from build123d import *


with BuildPart() as part:
    # Model → Повернуть1 (revolve)
    with BuildSketch(Plane.XY, mode=Mode.PRIVATE) as revolve_1_sk:
        Polygon((0, 0), (0, -22.297439151), (0.406986693, -22.5), (4.563171418, -22.5), (4.765560012, -22.297439151), (7.132579794, -17.847080181), (8.034078204, -18.53333859), (8.879510019, -18.045513069), (9.72476958, -18.601092135), (10.570023757, -18.045513069), (11.410266397, -18.530582514), (12.250724355, -18.045513069), (12.250724355, -17.741666414), (17.616266787, -17.741666414), (17.818865316, -17.539062501), (17.818865316, -16.425629172), (18.426031098, -16.425629172), (18.426031098, -17.387144556), (21.362129874, -17.387144556), (21.362129874, -16.425629172), (21.868225167, -16.425629172), (21.868225167, -17.493893941), (27.334902683, -17.493893941), (27.790688815, -18), (32.143900705, -18), (32.599331562, -17.544536845), (33.552402733, -17.544536845), (33.552338057, -16.75), (37.095113357, -16.75), (37.5, -16.425629172), (37.5, -12.801691559), (38.665364669, -12.801691559), (38.665364669, -13.294307916), (40.791343859, -13.294307916), (41.5, -12.586706835), (41.5, -10.75), (42.129406807, -10.75), (43.8, -9.548466361), (43.8, 0), align=None)
    revolve(revolve_1_sk.sketch.rotate(Axis((0, 0, 0), (1, 0, 0)), 270), axis=Axis((0, 0, 0), (1, 0, 0)))


solid = part.part
Part model, mm, in its own coordinate system. A direction names the side the tool comes from. Coordinates: 2 decimals unless noted, no trailing zeros. Write each loop counter-clockwise with the first axis right and the second up, starting at its lowest first coordinate (ties: lowest second). Pieces come first, ordered by that corner, then holes. Notation, with made-up numbers: (27, -32.5) - (41, -32.5) arc R27 cw to (41, -12.5) - close; hole circle Ø9 at (-1, 48). An arc over 180 degrees is marked (long way). Put each result on its own line as item: value.
1. Two-plate mould, pull along X, no slides. Class faces 1 (the cylindrical face through (38.09, -3.85, 12.21)), 2 (the cylindrical face through (29.998, -5.407, 17.169)), 3 (the flat face through (41.5, -5.7, 9.3)): +X half, -X half, draft (parallel to the pull), parting line (faces both ways), or undercut.
Final values:
face 1: undercut
face 2: draft
face 3: +X half
2. Flat gauge pins, fed straight in: pin 1 Ø1.5 at (x, y) = (15.5, -14) entering from -Z; pin 2 Ø10 at (x, z) = (10, 5) entering from -Y; pin 3 Ø17.5 at (y, z) = (-7, -2) entering from -X; pin 4 Ø3 at (x, z) = (4.5, 12.5) entering from +Y. Where does each tip first touch, or does it go through?
Final values:
pin 1: stops at z = -11.8
pin 2: stops at y = -21.34
pin 3: stops at x = 0
pin 4: stops at y = 19.63
3. Band-saw the part on B-B (x = 30). Write the cut outline in (y, z), then the cut area to 3 significant figures.
Final values:
outline: circle Ø36 at (0, 0)
area: 1,020 mm²
4. 3-axis set-ups, long thin cutter, end or side, ignore diameter. For faces 4 (the cylindrical face through (39.74, -13.18, -1.73)), 5 (the cylindrical face through (2.514, 8.618, 20.784)), 6 (the flat face through (21.362, 6.4, 15.4)): which of +Z, -Z, +X, -X, +Y, -Y reach the whole face in a straight line?
Final values:
face 4: +X
face 5: +X, -X
face 6: none
5. Probe line 1 along X through (y, z) = (12.5, -12); line 2 along X through (y, z) = (10, 12); line 3 along Y through (x, z) = (10.5, -7). List the from-to ranges inside material, lowest first. Write a range as [from, to].
Final values:
line 1: x = [0, 17.82], [18.43, 21.36], [21.87, 33.55]
line 2: x = [0, 37.5]
line 3: y = [-16.68, 16.68]
6. Band-saw the part on A-A (x = 14). Write the cut outline in (y, z), then the cut area to 3 significant figures.
Final values:
outline: circle Ø35.48 at (0, 0)
area: 989 mm²
